Verification items for the finished model (mm, model axes). A direction names the side the tool comes from. Give positions to 0.01 mm unless a question says otherwise; leave off trailing zeros. Write each loop counter-clockwise with the first axis right and the second up, starting at its lowest first coordinate (ties: lowest second). Pieces come first, ordered by that corner, then holes. Notation, with made-up numbers: (49, -7) -> (61, -7) arc R32 ccw to (61, 26) -> close; hole circle Ø1 at (-27.75, 9). An arc over 180 degrees is marked (long way). Answer as CSV lines item,"result". Start each with the question number.
1) Sectioned sample at A-A on x = 0. Record the cut outline in (y, z), and give its area (3 significant figures).
2) Tool access check on faces 4 (the flat face through (-5.46, -33.06, 3.76)), 5 (the flat face through (0, -23, 6.35)). Record the directions out of +Z, -Z, +X, -X, +Y, -Y that give a thin tool (end or side, any length) a straight path to the whole face; none if there is none.
3) Gauge pin test, flat ends, axial feed: pin 1 Ø5 at (x, y) = (2.5, -27.5) entering from -Z; pin 2 Ø1 at (y, z) = (-29.5, 6) entering from -X; pin 3 Ø1.5 at (x, z) = (4, 4.5) entering from +Y; pin 4 Ø1 at (x, y) = (0, -23) entering from -Z. Record the tip position at first contact, or that the pin passes through.
4) Mould release check, pull along Y, two halves, no side actions. Record for faces 1 (the cylindrical face through (-0.2, -24.5, 3.1)), 2 (the flat face through (0, -37, 0)), 3 (the cylindrical face through (0.06, -17.78, 3.76)): released by +Y, released by -Y, zero draft, split by the parting line, or undercut.
5) Material ranges on L1, parallel to Y at x = 0, z = 3.25; L2, parallel to Y at x = 0, z = 6.25; L3, parallel to X at y = -31, z = 5, recorded low to high.
6) Sectioned sample at C-C on z = 3. Give the number of separate pieces and of enclosed holes in the cut face, and give its area (3 significant figures).
7) Sectioned sample at B-B on y = -30.48. Record the cut outline in (x, z), and give its area (3 significant figures).
```python
from build123d import *

# Parameters (mm, degrees)
F1_DEPTH       = 7.62
F2_R           = 3.175
F4_D           = 2.7051
F6_D           = 4.4958
F6_CSINK_D     = 9.652
F6_CSINK_ANGLE = 82
F7_R           = 1.651
F8_DEPTH       = 7.621
F9_R           = 1.651
F10_DEPTH      = 1.27


with BuildPart() as f1:
    # F0 (on Top) → F1 (new body)
    with BuildSketch(Plane.XY):
        with BuildLine():
            Line((8.2333683595, -48.8408900969), (3.81, -17.3669888006))
            ThreePointArc((3.81, -17.3669888006), (0, -17.78), (-3.81, -17.3669888006))
            Line((-3.81, -17.3669888006), (-7.1361534431, -49.0132248892))
            ThreePointArc((-7.1361534431, -49.0132248892), (0.5553332003, -49.5268866883), (8.2333683595, -48.8408900969))
        make_face()
    extrude(amount=F1_DEPTH)

    # F2
    f2_edges = [f1.edges().sort_by_distance(p)[0] for p in [
        (-7.136153, -49.013225, 3.81),
        (-3.81, -17.366989, 3.81),
        (8.233368, -48.84089, 3.81),
        (3.81, -17.366989, 3.81),
    ]]
    fillet(f2_edges, radius=F2_R)

    # F4 (through all)
    with Locations(Plane.XY.offset(7.62)):
        with Locations((0, -46.4566)):
            Hole(F4_D / 2)

    # F6 (through all)
    with Locations(Plane.XY.offset(7.62)):
        with Locations((0, -30.48)):
            CounterSinkHole(F6_D / 2, F6_CSINK_D / 2, counter_sink_angle=F6_CSINK_ANGLE)

    # F7 (on face) → F8 (cut, through all)
    with BuildSketch(Plane(origin=(0, 0, 0), x_dir=(1, 0, 0), z_dir=(0, 0, -1))):
        with Locations((0, 22.86)):
            Circle(F7_R)
    extrude(amount=-F8_DEPTH, mode=Mode.SUBTRACT)

    # F9 (on face) → F10 (join)
    with BuildSketch(Plane.XY.offset(7.62)):
        with Locations((0, -22.86)):
            Circle(F9_R)
    extrude(amount=-F10_DEPTH)


solid = f1.part
```
Ans:
1,outline,"(-49.53, 0) -> (-47.81, 0) -> (-47.81, 7.62) -> (-49.53, 7.62) -> close; (-45.1, 0) -> (-32.73, 0) -> (-32.73, 4.65) -> (-35.31, 7.62) -> (-45.1, 7.62) -> close; (-28.23, 0) -> (-24.51, 0) -> (-24.51, 6.35) -> (-21.21, 6.35) -> (-21.21, 0) -> (-17.78, 0) -> (-17.78, 7.62) -> (-25.65, 7.62) -> (-28.23, 4.65) -> close"
1,area,"158 mm²"
2,face 4,"+Z, -Z, -X, +Y"
2,face 5,"-Z"
3,pin 1,"stops at z = 0"
3,pin 2,"stops at x = -5.14"
3,pin 3,"stops at y = -18.59"
3,pin 4,"stops at z = 6.35"
4,face 1,"undercut"
4,face 2,"zero draft"
4,face 3,"released by +Y"
5,L1,"y = -49.53 to -47.81, -45.1 to -32.73, -28.23 to -24.51, -21.21 to -17.78"
5,L2,"y = -49.53 to -47.81, -45.1 to -34.12, -26.84 to -24.51, -21.21 to -17.78"
5,L3,"x = -5.24 to -2.49, 2.49 to 5.73"
6,separate pieces,"1"
6,enclosed holes,"3"
6,area,"328 mm²"
7,outline,"(-5.19, 0) -> (-2.25, 0) -> (-2.25, 4.65) -> (-4.83, 7.62) -> (-5.19, 7.62) -> close; (2.25, 0) -> (5.65, 0) -> (5.65, 7.62) -> (4.83, 7.62) -> (2.25, 4.65) -> close"
7,area,"40.7 mm²"
